Check sheet for the drawn part. Datum: minimum x, y, z corner. Units: mm. Coordinates: 2 decimals unless noted, no trailing zeros. Loops run counter-clockwise (first coordinate to the right, second up) from the corner with the lowest first, then second, coordinate; pieces in that order, holes last. Notation, with made-up numbers: M -32,85 L 6,85 A21 cw 6,94 Z; hole C 24.25,-39 d2. An arc over 180 degrees is marked long. Use CSV: the item, a comma, the result in double quotes. Start each with the question number.
(1) Section check B-B on z = 115.5. Record the cut outline in (x, y).
(2) Section check C-C on z = 41. Record the cut outline in (x, y).
(3) Scan lines: line 1 (Z direction, x = 0.9, y = 5.8); line 2 (Y direction, x = 0.55, z = 155.5); line 3 (Z direction, x = 7, y = 24.5). Record each from-to range of solid material in increasing order.
(4) Section check A-A on x = 8.75. Record the cut outline in (y, z).
(5) Draft check along Z on the marked faces 1, 2 and 3. Enter one of: pulls with the +Z half, pulls with the -Z half, needs draft (parallel to the pull), parting line crosses it, or undercut.
(6) Go/stop test with flat-tipped pins: pin 1 Ø3 at (y, z) = (46.5, 97) entering from +X; pin 2 Ø3 at (x, z) = (11.5, 65.5) entering from +Y; pin 3 Ø1.2 at (x, y) = (16.5, 33) entering from -Z. Record where each tip stops, or that it passes through.
(7) Section check D-D on z = 24. Record the cut outline in (x, y), and give its area (3 significant figures).
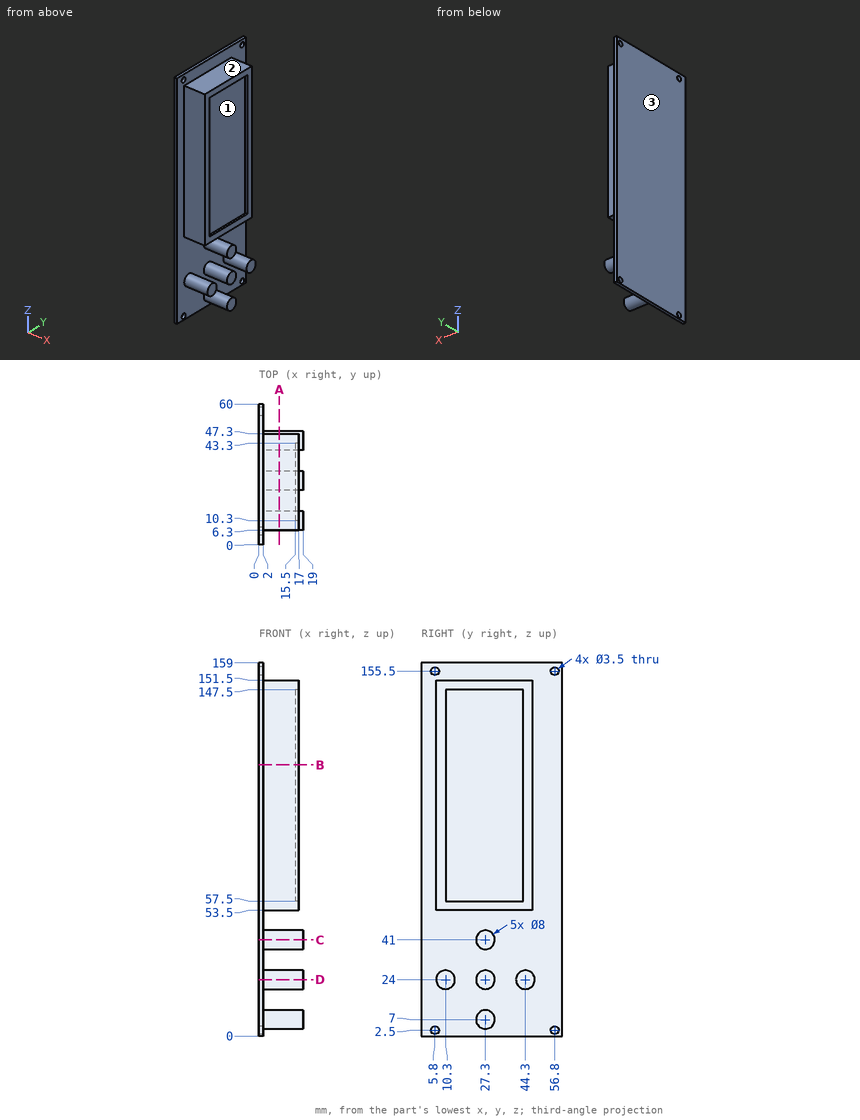
Outcome:
1,outline,"M 0,0 L 2,0 L 2,6.3 L 17,6.3 L 17,10.3 L 15.5,10.3 L 15.5,43.3 L 17,43.3 L 17,47.3 L 2,47.3 L 2,60 L 0,60 Z"
2,outline,"M 0,0 L 2,0 L 2,23.3 L 19,23.3 L 19,31.3 L 2,31.3 L 2,60 L 0,60 Z"
3,line 1,"z = 0 to 0.75, 4.25 to 153.75, 157.25 to 159"
3,line 2,"y = 0 to 4.05, 7.55 to 55.05, 58.55 to 60"
3,line 3,"z = 4.14 to 9.86, 21.14 to 26.86, 38.14 to 43.86, 53.5 to 151.5"
4,outline,"C 10.3,24 d8; M 6.3,53.5 L 47.3,53.5 L 47.3,151.5 L 6.3,151.5 Z; C 27.3,7 d8; C 27.3,24 d8; C 27.3,41 d8; C 44.3,24 d8"
5,face 1,"undercut"
5,face 2,"pulls with the +Z half"
5,face 3,"needs draft"
6,pin 1,"stops at x = 17"
6,pin 2,"stops at y = 47.3"
6,pin 3,"stops at z = 53.5"
7,outline,"M 0,0 L 2,0 L 2,6.3 L 19,6.3 L 19,14.3 L 2,14.3 L 2,23.3 L 19,23.3 L 19,31.3 L 2,31.3 L 2,40.3 L 19,40.3 L 19,48.3 L 2,48.3 L 2,60 L 0,60 Z"
7,area,"528 mm²"
